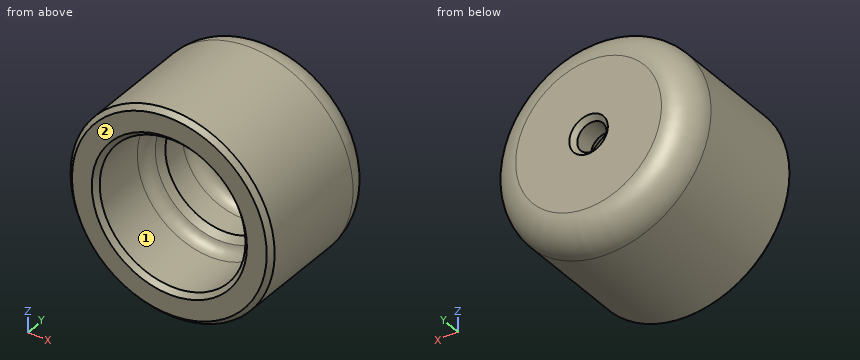
```python
from build123d import *

# Parameters (mm, degrees)
FILLET1_R = 1.5875
FILLET2_R = 3.175


with BuildPart() as part:
    # Sketch1 → Revolve1 (revolve)
    with BuildSketch(Plane.XY, mode=Mode.PRIVATE) as revolve1_sk:
        Polygon((1.5875, 15.875), (1.5875, 12.7), (6.35, 12.7), (6.35, 7.9375), (7.9375, 7.9375), (7.9375, 0), (11.1125, 0), (11.1125, 15.875), align=None)
    revolve(revolve1_sk.sketch.rotate(Axis((0, 3.137063419, 0), (0, -1, 0)), 90), axis=Axis((0, 3.137063419, 0), (0, -1, 0)))

    # Fillet1
    fillet1_edges = [part.edges().sort_by_distance(p)[0] for p in [
        (0, 7.9375, -7.9375),
        (0, 12.7, -6.35),
    ]]
    fillet(fillet1_edges, radius=FILLET1_R - 0.0001)  # a hair under: the kernel refuses the full size

    # Fillet2
    fillet2_edges = [part.edges().sort_by_distance(p)[0] for p in [
        (0, 15.875, -11.1125),
    ]]
    fillet(fillet2_edges, radius=FILLET2_R)

    # Chamfer1: read off the stored shape, not the designer's step
    # Chamfer1 outline → Chamfer1 (revolve, cut)
    with BuildSketch(Plane.XY):
        Polygon((1.5875, 15.875), (1.5875, 15.367), (2.0955, 15.875), align=None)
        Polygon((2.0955, 12.7), (1.5875, 13.208), (1.5875, 12.7), align=None)
        Polygon((6.994887663, 7.800612337), (6.35, 8.4455), (6.35, 7.800612337), align=None)
        Polygon((8.4455, 0), (7.9375, 0.508), (7.9375, 0), align=None)
        Polygon((11.1125, 0.508), (10.6045, 0), (11.1125, 0), align=None)
    revolve(axis=Axis((0, 0, 0), (0, 1, 0)), mode=Mode.SUBTRACT)


solid = part.part
```
The listing builds one solid part. Answer for the finished solid, in the listing's coordinates (mm). Face numbers are marked on the shaded views. A direction names the side the tool comes from. Round coordinates to 2 decimals unless told otherwise and drop trailing zeros. Write each loop counter-clockwise with the first axis right and the second up, starting at its lowest first coordinate (ties: lowest second). Pieces come first, ordered by that corner, then holes. Notation, with made-up numbers: (-20, -31.5) -> (-14, -31.5) arc R25 cw to (-14, 6.5) -> close; hole circle Ø3 at (44, 34.5). An arc over 180 degrees is marked (long way). Use CSV: the item, a comma, the result in double quotes. Start each with the question number.
(1) Section D-D on y = 3 is taken. Give the vertices of the cut face in (x, z) (1 decimal), then the cut area to 3 significant figures.
(2) Each of these flat-tipped pins is pushed along its axis until it touches: pin 1 (6 mm diameter, centred on x = 4.5, y = 7, fed in from +Z); pin 2 (9.5 mm diameter, centred on x = 0, z = 0, fed in from -Y); pin 3 (7.5 mm diameter, centred on x = -1, z = 2, fed in from -Y). Where does it stop, or does it pass through?
(3) Consider L1, parallel to X at y = 3.15, z = 0; L2, parallel to X at y = 10.35, z = 0; L3, parallel to Z at x = -6, y = 1. Determine where each line is inside the solid, lowest interval first. Write a range as from..to.
(4) Which of the six approach directions +Z, -Z, +X, -X, +Y, -Y give full straight-line access (tool end or side, diameter ignored) to the marked faces 1 and 2?
A:
1,outline,"circle Ø22.2 at (0, 0); hole circle Ø15.9 at (0, 0)"
1,area,"190 mm²"
2,pin 1,"stops at z = 11.01"
2,pin 2,"stops at y = 12.7"
2,pin 3,"stops at y = 12.12"
3,L1,"x = -11.11..-7.94, 7.94..11.11"
3,L2,"x = -11.11..-6.35, 6.35..11.11"
3,L3,"z = -9.35..-5.2, 5.2..9.35"
4,face 1,"-Y"
4,face 2,"+Z, -Z, +X, -X, -Y"
